For this review, take the finished solid that the model builds, in its own axes (mm). A direction names the side the tool comes from. Round coordinates to 2 decimals unless told otherwise and drop trailing zeros. Write each loop counter-clockwise with the first axis right and the second up, starting at its lowest first coordinate (ties: lowest second). Pieces come first, ordered by that corner, then holes. Notation, with made-up numbers: (28, 71.25) -> (67, 71.25) arc R26 ccw to (67, 104.25) -> close; hole circle Ø10 at (-7.5, 71.25). An arc over 180 degrees is marked (long way). Write each question's results on one line, items separated by ' | '. Start each with the question number.
Item 1: Add section A-A (y = 19). Count the separate pieces of the cut face and the enclosed holes in it, plus the area to 3 significant figures.
Item 2: Add section D-D (z = 71). State the section outline as (x, y) points.
Item 3: To check wall thickness, follow line 1 along X through (y, z) = (45, 1.5); line 2 along X through (y, z) = (40.5, -13.5); line 3 along Z through (x, y) = (28.5, 45). State the ranges of each line that lie inside material, in increasing order.
Item 4: The part is to be moulded in two halves that separate along Z. For faces 3 (the flat face through (-35.76, 25.04, 22.72)), 4 (the cylindrical face through (296.314, 25.044, -1.027)), 5 (the flat face through (-40.06, 25.04, -13.8)), 6 (the flat face through (104, 0, 1)), say which applies: +Z half, -Z half, draft (parallel to the pull), parting line (faces both ways), or undercut.
Item 5: Clearance check with flat-ended pins moving along their axes: pin 1 (6 mm diameter, centred on y = 17.5, z = 11.5, fed in from +X); pin 2 (8 mm diameter, centred on x = 82, z = 11.5, fed in from -Y); pin 3 (12 mm diameter, centred on y = 5.5, z = 51.5, fed in from +X); pin 4 (3 mm diameter, centred on y = 35, z = -7, fed in from -X). State where each tip first meets the part, or that it passes through.
Item 6: Add section C-C (x = 34). State the section outline as (y, z) points.
Item 7: Tool access review of faces 1 (the flat face through (-4.538, 25.044, 42.125)), 2 (the flat face through (104, 50.8, 1)): name each direction out of +Z, -Z, +X, -X, +Y, -Y from which nothing blocks a thin tool from reaching the whole face with its end or side.
Item 8: Add section B-B (z = -8). State the section outline as (x, y) points.
from build123d import *

# Parameters (mm, degrees)
F1_DEPTH = 50.8


# Not quite as in the source:
# - a feature names something its author has since deleted; it is built from what else it names


with BuildPart() as f1:
    # F0 (on Front) → F1 (new body)
    with BuildSketch(Plane.XZ):
        with BuildLine():
            Line((20.7350080501, 79.903453875), (0, 82.55))
            ThreePointArc((0, 82.55), (-82.55, 0), (0, -82.55))
            Line((0, -82.55), (20.7350080501, -79.903453875))
            ThreePointArc((20.7350080501, -79.903453875), (65.2923326836, -50.511521386), (82.55, 0))
            ThreePointArc((82.55, 0), (65.2923326836, 50.511521386), (20.7350080501, 79.903453875))
        make_face()
        Polygon((44.563520115, 15.0143387373), (39.5235830399, -25.4798759112), (4.7215818015, -46.7872243038), (-33.6358668361, -32.8628385102), (-46.6648216995, 5.8079349613), (-24.5542140343, 40.1052149467), (16.0462176134, 44.2024500799), align=None, mode=Mode.SUBTRACT)
        with BuildLine():
            ThreePointArc((20.7350080501, 79.903453875), (10.4516119, 81.8856905002), (0, 82.55))
            Line((0, 82.55), (20.7350080501, 79.903453875))
        make_face()
        with BuildLine():
            Line((20.7350080501, -79.903453875), (0, -82.55))
            ThreePointArc((0, -82.55), (10.4516119, -81.8856905002), (20.7350080501, -79.903453875))
        make_face()
        with BuildLine():
            Line((251.9559707698, 50.391194154), (20.7350080501, 79.903453875))
            ThreePointArc((20.7350080501, 79.903453875), (65.2923326836, 50.511521386), (82.55, 0))
            ThreePointArc((82.55, 0), (65.2923326836, -50.511521386), (20.7350080501, -79.903453875))
            Line((20.7350080501, -79.903453875), (251.9559707698, -50.391194154))
            ThreePointArc((251.9559707698, -50.391194154), (194.7242096006, 0), (251.9559707698, 50.391194154))
        make_face()
        with BuildLine():
            ThreePointArc((296.3242096006, 0), (283.6514535831, 33.5701246096), (251.9559707698, 50.391194154))
            ThreePointArc((251.9559707698, 50.391194154), (194.7242096006, 0), (251.9559707698, -50.391194154))
            ThreePointArc((251.9559707698, -50.391194154), (283.6514535831, -33.5701246096), (296.3242096006, 0))
        make_face()
        Polygon((273.0559987523, 19.6265456703), (276.2871913154, -14.0299559819), (248.7554021637, -33.6565016521), (217.9924204489, -19.6265456703), (214.7612278858, 14.0299559819), (242.2930170375, 33.6565016521), align=None, mode=Mode.SUBTRACT)
    extrude(amount=-F1_DEPTH)


solid = f1.part
Responses:
1) separate pieces: 1 | enclosed holes: 2 | area: 38,600 mm^2
2) outline: (-42.11, 0) -> (90.49, 0) -> (90.49, 50.8) -> (-42.11, 50.8) -> close
3) line 1: x = -82.54 to -45.21, 42.88 to 215.96, 274.8 to 296.3 | line 2: x = -81.44 to -40.16, 41.01 to 217.4, 276.24 to 294.5 | line 3: z = -78.91 to -32.23, 31.46 to 78.91
4) face 3: undercut | face 4: parting line | face 5: undercut | face 6: draft
5) pin 1: stops at x = 295.61 | pin 2: stops at y = 0 | pin 3: stops at x = 268.12 | pin 4: stops at x = -82.37
6) outline: (0, -78.21) -> (50.8, -78.21) -> (50.8, -28.86) -> (0, -28.86) -> close; (0, 25.83) -> (50.8, 25.83) -> (50.8, 78.21) -> (0, 78.21) -> close
7) face 1: +Y, -Y | face 2: +Z, -Z, +X, -X, +Y
8) outline: (-82.16, 0) -> (-42.01, 0) -> (-42.01, 50.8) -> (-82.16, 50.8) -> close; (41.7, 0) -> (216.88, 0) -> (216.88, 50.8) -> (41.7, 50.8) -> close; (275.71, 0) -> (295.69, 0) -> (295.69, 50.8) -> (275.71, 50.8) -> close
